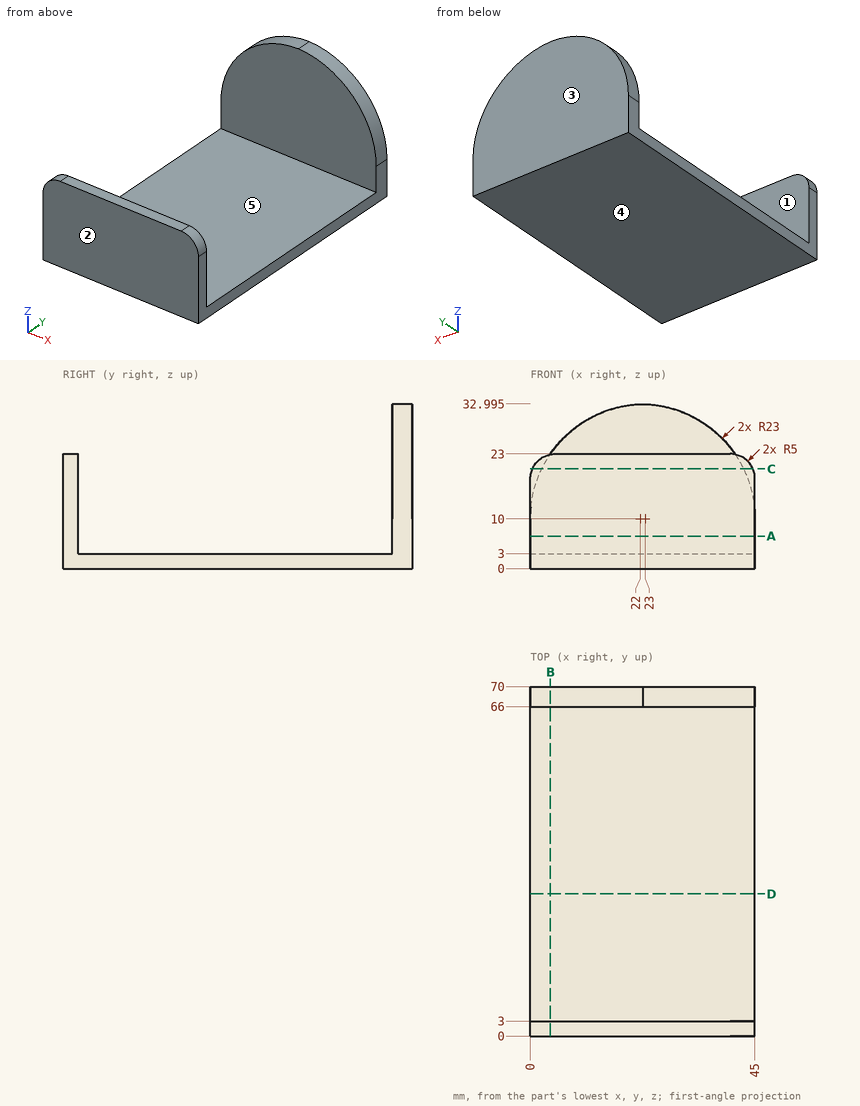
Job drawing, mm, ordinate dimensions from the low corner. One solid piece. A direction names the side the tool comes from. Coordinates: 2 decimals unless noted, no trailing zeros. Order: outer loops, then holes, each group sorted by start corner. A loop starts at its lowest first (then second) coordinate and runs counter-clockwise, first axis right, second up. Notation, with made-up numbers: (-4, 75) -> (10, 75) arc R9 ccw to (10, 87) -> close; hole circle Ø6 at (39, -4). An arc over 180 degrees is marked (long way). Put each result on its own line as item: value. Start each with the question number.
(1) Which spindle directions (+Z, -Z, +X, -X, +Y, -Y) get a long thin tool onto all of the face, cutting with end or side? Do the marked faces 4 and 5. Say none if no direction does.
(2) Mould opens along Y. For the marked faces 1, 2 and 3 say: pulls with the +Y half, pulls with the -Y half, needs draft (parallel to the pull), parting line crosses it, or undercut.
(3) Band-saw the part on B-B (x = 4). Give the cut face in (y, z).
(4) Probe line 1 along Y through (x, z) = (26, 5); line 2 along Z through (x, y) = (35, 10.5); line 3 along Y through (x, z) = (17.5, 28.5). List the from-to ranges inside material, lowest first. Write a range as [from, to].
(5) Band-saw the part on C-C (z = 20). Give the cut face in (x, y).
(6) Pin check, flat tips, straight feed: pin 1 Ø10 at (x, z) = (7.5, 20) entering from -Y; pin 2 Ø13.5 at (x, y) = (32, 30.5) entering from +Z; pin 3 Ø3.5 at (x, y) = (25.5, 2) entering from +Z. Stop position of each tip, or through.
(7) Band-saw the part on A-A (z = 6.5). Give the cut face in (x, y).
(8) Band-saw the part on D-D (y = 28.5). Give the cut face in (x, z), then the cut area to 3 significant figures.
Determined:
1. face 4: -Z, +X, -X, +Y, -Y
1. face 5: +Z, +X, -X
2. face 1: undercut
2. face 2: pulls with the -Y half
2. face 3: pulls with the +Y half
3. outline: (0, 0) -> (70, 0) -> (70, 22.96) -> (66, 22.96) -> (66, 3) -> (3, 3) -> (3, 22.9) -> (0, 22.9) -> close
4. line 1: y = [0, 3], [66, 70]
4. line 2: z = [0, 3]
4. line 3: y = [66, 70]
5. outline: (0.42, 0) -> (44.58, 0) -> (44.58, 3) -> (0.42, 3) -> close; (2.29, 66) -> (42.71, 66) -> (42.71, 70) -> (2.29, 70) -> close
6. pin 1: stops at y = 0
6. pin 2: stops at z = 3
6. pin 3: stops at z = 23
7. outline: (0, 0) -> (45, 0) -> (45, 3) -> (0, 3) -> close; (0, 66) -> (45, 66) -> (45, 70) -> (0, 70) -> close
8. outline: (0, 0) -> (45, 0) -> (45, 3) -> (0, 3) -> close
8. area: 135 mm²
